Source: three-view drawing plus pictorial views. Frame: mm from the lowest corner of the part. A direction names the side the tool comes from. Coordinates: 2 decimals unless noted, no trailing zeros. Write each loop counter-clockwise with the first axis right and the second up, starting at its lowest first coordinate (ties: lowest second). Pieces come first, ordered by that corner, then holes. Notation, with made-up numbers: (-33, 56) - (-26, 56) arc R13 cw to (-26, 63) - close; hole circle Ø3 at (-17.5, 71.5). An arc over 180 degrees is marked (long way). Put each result on its own line as item: value.
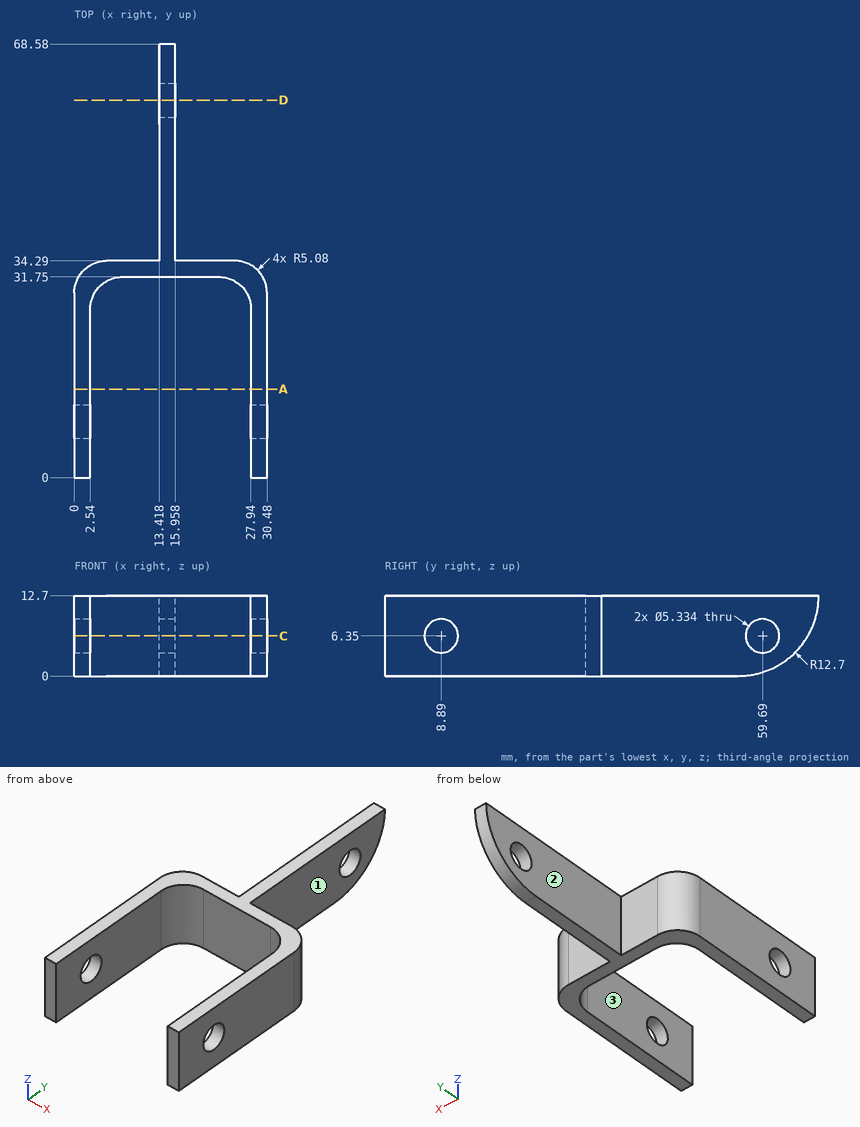
1. Set-up query: the marked faces 1, 2 and 3. Return all of +Z, -Z, +X, -X, +Y, -Y with unobstructed straight access to the full face (end or side cutting, diameter ignored); none if empty.
Answer below:
face 1: +Z, -Z, +X, +Y
face 2: +Z, -Z, -X, +Y
face 3: +Z, -Z, -Y
2. Section query C-C (z = 6.35). Return loops of the section in (x, y), then the cut area to 3 significant figures.
Answer below:
outline: (0, 0) - (2.54, 0) - (2.54, 6.22) - (0, 6.22) - close; (0, 11.56) - (2.54, 11.56) - (2.54, 26.67) arc R5.08 cw to (7.62, 31.75) - (22.86, 31.75) arc R5.08 cw to (27.94, 26.67) - (27.94, 11.56) - (30.48, 11.56) - (30.48, 29.21) arc R5.08 ccw to (25.4, 34.29) - (15.96, 34.29) - (15.96, 57.02) - (13.42, 57.02) - (13.42, 34.29) - (5.08, 34.29) arc R5.08 ccw to (0, 29.21) - close; (13.42, 62.36) - (15.96, 62.36) - (15.96, 66.88) - (13.42, 66.88) - close; (27.94, 0) - (30.48, 0) - (30.48, 6.22) - (27.94, 6.22) - close
area: 281 mm²
3. Section query A-A (y = 14). Return loops of the section in (x, z), then the cut area to 3 significant figures.
Answer below:
outline: (0, 0) - (2.54, 0) - (2.54, 12.7) - (0, 12.7) - close; (27.94, 0) - (30.48, 0) - (30.48, 12.7) - (27.94, 12.7) - close
area: 64.5 mm²
4. Section query D-D (y = 59.69). Return loops of the section in (x, z) (1 decimal).
Answer below:
outline: (13.4, 0.6) - (16, 0.6) - (16, 3.7) - (13.4, 3.7) - close; (13.4, 9) - (16, 9) - (16, 12.7) - (13.4, 12.7) - close
5. Pin query (flat end, axial travel): pin 1 Ø4.5 at (x, z) = (22.5, 3.5) entering from +Y; pin 2 Ø3 at (y, z) = (54.5, 2.5) entering from -X; pin 3 Ø1 at (x, z) = (4, 5) entering from -Y. Return the tip coordinate at first contact, or that it passes through.
Answer below:
pin 1: stops at y = 34.29
pin 2: stops at x = 13.42
pin 3: stops at y = 29.64
6. Ray query, probe 1 along Z at (x, y) = (1, 8.89); probe 2 along X at (y, z) = (22, 1.75); probe 3 along X at (y, z) = (64, 9.25). Return the intervals inside material, ascending. Write a range as from..to.
Answer below:
probe 1: z = 0..3.68, 9.02..12.7
probe 2: x = 0..2.54, 27.94..30.48
probe 3: x = 13.42..15.96
